from build123d import *

# Parameters (mm, degrees)
SKETCH1_W           = 20
SKETCH1_H           = 0.25
BOSS_EXTRUDE1_DEPTH = 2
SKETCH2_W           = 0.25
SKETCH2_H           = 5.5
BOSS_EXTRUDE2_DEPTH = 3.5
FILLET1_R           = 0.25
FILLET2_R           = 1.75
BOSS_EXTRUDE3_START = -2.25
SKETCH3_R           = 0.75
BOSS_EXTRUDE3_DEPTH = 2.5
BOSS_EXTRUDE5_DEPTH = 3
FILLET3_R           = 1.5
FILLET4_R           = 0.25


with BuildPart() as part:
    # Sketch1 → Boss-Extrude1 (new, symmetric)
    with BuildSketch(Plane.XY):
        Rectangle(SKETCH1_W, SKETCH1_H)
    extrude(amount=BOSS_EXTRUDE1_DEPTH, both=True)

    # Sketch2 → Boss-Extrude2 (add)
    with BuildSketch(Plane(origin=(10, 0, 0), x_dir=(0, 0, -1), z_dir=(1, 0, 0))):
        with Locations((-2.125, 2.625)):
            Rectangle(SKETCH2_W, SKETCH2_H)
        with Locations((2.125, 2.625)):
            Rectangle(SKETCH2_W, SKETCH2_H)
    extrude(amount=-BOSS_EXTRUDE2_DEPTH)

    # Fillet1
    fillet1_edges = [part.edges().sort_by_distance(p)[0] for p in [
        (8.25, -0.125, -2.25),
        (8.25, -0.125, 2.25),
        (8.25, 0.125, -2),
        (8.25, 0.125, 2),
    ]]
    fillet(fillet1_edges, radius=FILLET1_R)

    # Fillet2
    fillet2_edges = [part.edges().sort_by_distance(p)[0] for p in [
        (10, 5.375, -2.125),
        (6.5, 5.375, -2.125),
        (6.5, 5.375, 2.125),
        (10, 5.375, 2.125),
    ]]
    fillet(fillet2_edges, radius=FILLET2_R - 0.0001)  # a hair under: the kernel refuses the full size

    # Sketch3 → Boss-Extrude3 (add, symmetric)
    with BuildSketch(Plane.XY.offset(2.25).offset(BOSS_EXTRUDE3_START)):
        with Locations(Location((8.25, 3.625, 0), (0, 0, 180))):
            Circle(SKETCH3_R)
    extrude(amount=BOSS_EXTRUDE3_DEPTH, both=True)

    # Sketch5 → Boss-Extrude5 (add)
    with BuildSketch(Plane.ZY.offset(10)):
        Polygon((-2, -0.125), (-2.75, -0.125), (-2.75, -3.375), (-3, -3.375), (-3, 0.125), (-2, 0.125), align=None)
        Polygon((3, 0.125), (2, 0.125), (2, -0.125), (2.75, -0.125), (2.75, -3.375), (3, -3.375), align=None)
    extrude(amount=-BOSS_EXTRUDE5_DEPTH)

    # Fillet3
    fillet3_edges = [part.edges().sort_by_distance(p)[0] for p in [
        (-10, -3.375, 2.875),
        (-7, -3.375, 2.875),
        (-7, -3.375, -2.875),
        (-10, -3.375, -2.875),
    ]]
    fillet(fillet3_edges, radius=FILLET3_R - 0.0001)  # a hair under: the kernel refuses the full size

    # Fillet4
    fillet4_edges = [part.edges().sort_by_distance(p)[0] for p in [
        (-8.5, -0.125, -2.75),
        (-8.5, 0.125, -3),
        (-8.5, 0.125, 3),
        (-8.5, -0.125, 2.75),
    ]]
    fillet(fillet4_edges, radius=FILLET4_R)


solid = part.part
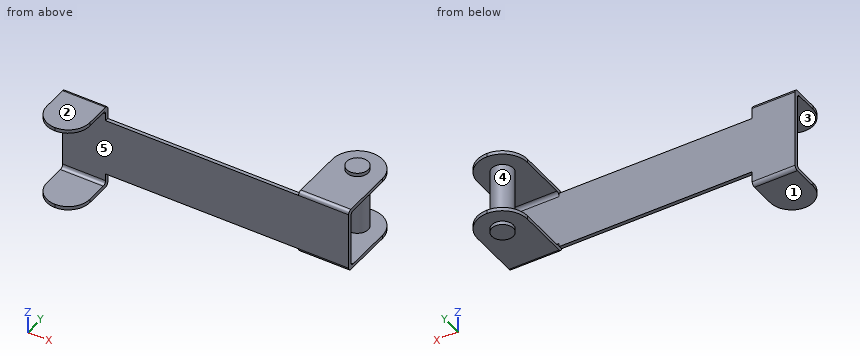
Design review of the part built by this model. Coordinates are the model's own, in mm. Face numbers are marked on the shaded views. A direction names the side the tool comes from. Round coordinates to 2 decimals unless told otherwise and drop trailing zeros. Write each loop counter-clockwise with the first axis right and the second up, starting at its lowest first coordinate (ties: lowest second). Pieces come first, ordered by that corner, then holes. Notation, with made-up numbers: (45, 50.5) - (93, 50.5) arc R19 ccw to (93, 84.5) - close; hole circle Ø8 at (-17.75, 58). An arc over 180 degrees is marked (long way). Use a Markdown table: item, result. Add a question column.
1. We need section B-B (y = 2.25). State the section outline as (x, z) points, then the cut area to 3 significant figures.
2. Mouldability with a two-part tool opening along Z and no side actions: class the marked faces 1, 2 and 3 as +Z half, -Z half, draft (parallel to the pull), parting line (faces both ways), or undercut.
3. For the marked faces 4 and 5, list the 3-axis set-ups (+Z, -Z, +X, -X, +Y, -Y) from which the entire face can be reached by the end or side of a thin tool; tool diameter is ignored.
4. Clearance check with flat-ended pins moving along their axes: pin 1 (4 mm diameter, centred on x = 7.5, y = 2, fed in from +Z); pin 2 (3 mm diameter, centred on x = -2.5, y = 0, fed in from +Z); pin 3 (1.5 mm diameter, centred on x = 1.5, z = 0, fed in from -Y) (3 decimals). State where each tip first meets the part, or that it passes through.
5. We need section A-A (y = -1.25). State the section outline as (x, z) points.
6. We need section D-D (x = -1.5). State the section outline as (y, z) points (3 decimals).
7. Wall thickness on probe 1 along Y at (x, z) = (-4.75, -1.9) (3 decimals); probe 2 along Z at (x, y) = (7.75, 0.25); probe 3 along X at (y, z) = (4, 0.1): over which ranges is each line inside the solid? List them lowest first.
8. We need section C-C (z = -0.15). State the section outline as (x, y) points (3 decimals).
Output:
| question | item | result |
|---|---|---|
| 1 | outline | (6.5, -2.25) - (10, -2.25) - (10, -2) - (6.5, -2) - close; (6.5, 2) - (10, 2) - (10, 2.25) - (6.5, 2.25) - close |
| 1 | area | 1.75 mm2 |
| 2 | face 1 | -Z half |
| 2 | face 2 | +Z half |
| 2 | face 3 | undercut |
| 3 | face 4 | none |
| 3 | face 5 | +X, -X, -Y |
| 4 | pin 1 | stops at z = 2.5 |
| 4 | pin 2 | stops at z = 2 |
| 4 | pin 3 | stops at y = -0.125 |
| 5 | outline | (-10, -3) - (-7, -3) - (-7, -2.75) - (-10, -2.75) - close; (-10, 2.75) - (-7, 2.75) - (-7, 3) - (-10, 3) - close |
| 6 | outline | (-0.125, -2) - (0.125, -2) - (0.125, 2) - (-0.125, 2) - close |
| 7 | probe 1 | y = -0.125 to 0.125 |
| 7 | probe 2 | z = -2.25 to -1.97, 1.97 to 2.25 |
| 7 | probe 3 | x = 7.6 to 8.9 |
| 8 | outline | (-10, -0.125) - (10, -0.125) - (10, 0.125) - (-10, 0.125) - close; circle Ø1.5 at (8.25, 3.625) |
